Can you work these out from the model? Positions are in its coordinate system, mm. A direction names the side the tool comes from. Give positions to 0.01 mm unless a question says otherwise; leave off trailing zeros. Loops run counter-clockwise (first coordinate to the right, second up) from the corner with the lowest first, then second, coordinate; pieces in that order, holes last. Notation, with made-up numbers: (10.25, 71.5) - (58.25, 71.5) arc R11 cw to (58.25, 79.5) - close; hole circle Ø6 at (21.5, 24.25). An arc over 180 degrees is marked (long way). Answer in a Markdown table with one row per item.
Autodesk Inventor part; units mm, degrees
ref_plane "Work Plane1" through (0, 0, 10) normal (0, 0, 1) x (1, 0, 0)
ref_plane "YZ Plane" through (0, 0, 0) normal (1, 0, 0) x (0, 1, 0)
ref_plane "XZ Plane" through (0, 0, 0) normal (0, 1, 0) x (-1, 0, 0)
ref_plane "Work Plane1" through (0, 0, 10) normal (0, 0, 1) x (1, 0, 0)
sketch "Sketch1" plane through (0, 0, 10) normal (0, 0, 1) x (1, 0, 0)
  line L0 (-4.0299, -0.3538) -> (-2.2322, 1.4439) construction
  arc A0 (-1.4439, 2.2322) -> (-2.2322, 1.4439) centre (-0.9299, 0.9299) ccw construction
  line L1 (-1.4439, 2.2322) -> (0.3538, 4.0299) construction
  line L2 (-37.8299, 42.8299) -> (-37.8299, 37.8299) construction
  line L3 (-37.8299, 37.8299) -> (-42.9208, 37.8299) construction
  line L4 (-37.8299, 42.2137) -> (-37.8299, 45.8299) construction
  line L5 (-37.8299, 45.8299) -> (-4.0299, 45.8299) construction
  line L6 (-4.0299, 45.8299) -> (-4.0299, 42.2137) construction
  line L7 (-4.0299, 4.0299) -> (0.3538, 4.0299)
  circle A1 centre (-20.9299, 20.9299) radius 17.5
  line L8 (-20.9299, 58.9723) -> (17.1124, 20.9299) construction
  line L9 (17.1124, 20.9299) -> (-20.9299, -17.1124) construction
  line L10 (-20.9299, -17.1124) -> (-58.9723, 20.9299) construction
  line L11 (-58.9723, 20.9299) -> (-20.9299, 58.9723) construction
  line L12 (-20.9299, 58.9723) -> (-20.9299, -17.1124) construction
  line L13 (17.1124, 20.9299) -> (-58.9723, 20.9299) construction
  line L14 (-20.9299, 58.9723) -> (32.8701, 58.9723) construction
  line L15 (-43.4299, 43.4299) -> (1.5701, 43.4299) construction
  line L16 (1.5701, 43.4299) -> (1.5701, -1.5701) construction
  line L17 (1.5701, -1.5701) -> (-43.4299, -1.5701) construction
  line L18 (-43.4299, -1.5701) -> (-43.4299, 43.4299) construction
  line L19 (-43.4299, 43.4299) -> (1.5701, -1.5701) construction
  line L20 (1.5701, 43.4299) -> (-43.4299, -1.5701) construction
  line L21 (-43.4299, 5.3876) -> (-43.4299, 36.4723)
  line L22 (-43.4299, 36.4723) -> (-36.4723, 43.4299)
  line L23 (-36.4723, 43.4299) -> (-5.3876, 43.4299)
  line L24 (-5.3876, 43.4299) -> (1.5701, 36.4723)
  line L25 (1.5701, 36.4723) -> (1.5701, 5.3876)
  line L26 (1.5701, 5.3876) -> (-5.3876, -1.5701)
  line L27 (-5.3876, -1.5701) -> (-36.4723, -1.5701)
  line L28 (-36.4723, -1.5701) -> (-43.4299, 5.3876)
  line L29 (-4.0299, 42.2137) -> (-37.8299, 42.2137)
  line L30 (-4.0299, -0.3538) -> (-4.0299, 4.0299)
  circle A2 centre (-20.9299, 20.9299) radius 1.5
  line L31 (-10.9299, 10.9299) -> (-30.9299, 10.9299) construction
  line L32 (-30.9299, 10.9299) -> (-30.9299, 30.9299) construction
  line L33 (-30.9299, 30.9299) -> (-10.9299, 30.9299) construction
  line L34 (-10.9299, 30.9299) -> (-10.9299, 10.9299) construction
  line L35 (-10.9299, 10.9299) -> (-30.9299, 30.9299) construction
  line L36 (-30.9299, 10.9299) -> (-10.9299, 30.9299) construction
  circle A3 centre (-30.9299, 30.9299) radius 1.4
  circle A4 centre (-30.9299, 10.9299) radius 1.4
  circle A5 centre (-10.9299, 10.9299) radius 1.4
  line L37 (-45.8299, 37.8299) -> (-42.0723, 37.8299) construction
  line L38 (-42.1723, 37.7299) -> (-45.8299, 37.7299)
  line L39 (-45.8299, 37.7299) -> (-45.8299, 4.1299)
  line L40 (-45.8299, 4.1299) -> (-42.1723, 4.1299)
  line L41 (-42.1723, 4.1299) -> (-42.1723, 37.7299)
  line L42 (-45.8299, 4.0299) -> (-42.0723, 4.0299) construction
  line L43 (-45.8299, 37.8299) -> (-42.0723, 37.8299)
  line L44 (-37.7299, 45.8299) -> (-4.1299, 45.8299)
  line L45 (-4.1299, 45.8299) -> (-4.1299, 42.1723)
  line L46 (-4.1299, 42.1723) -> (-37.7299, 42.1723)
  line L47 (-37.7299, 42.1723) -> (-37.7299, 45.8299)
  line L48 (0.4701, 37.8299) -> (0.4701, 4.0299) construction
  line L49 (0.4701, 4.0299) -> (3.9701, 4.0299) construction
  line L50 (3.9701, 37.8299) -> (3.9701, 4.0299) construction
  line L51 (0.4701, 37.8299) -> (3.9701, 37.8299) construction
  line L52 (-45.8299, -3.9701) -> (-4.0299, -3.9701) construction
  line L53 (0.3124, 37.7299) -> (3.9701, 37.7299)
  line L54 (3.9701, 37.7299) -> (3.9701, 4.1299)
  line L55 (3.9701, 4.1299) -> (0.3124, 4.1299)
  line L56 (0.3124, 4.1299) -> (0.3124, 37.7299)
  line L57 (-4.1713, -0.3538) -> (-37.7299, -0.3538)
  line L58 (-37.7299, -0.3538) -> (-37.7299, -3.9701)
  line L59 (-37.7299, -3.9701) -> (-4.1713, -3.9701)
  line L60 (-4.1713, -3.9701) -> (-4.1713, -0.3538)
  point P0 (-37.8299, 4.0299)
  dimension "d18" = 53.8
  dimension "d19" = 45
  dimension "d20" = 53.8
  dimension "d21" = 45
  dimension "d22" = 45
  dimension "d30" = 20
  dimension "d31" = 20
  dimension "d32" = 2.8
  dimension "d33" = 2.8
  dimension "d34" = 2.8
  dimension "d35" = 3
  dimension "d36" = 0.1
  dimension "d37" = 0.1
  dimension "d38" = 0.1
  dimension "d39" = 0.1
extrude "Extrusion1" add sketch "Sketch1" along normal blind 3 contours L30 L26 L57 L28 L41 L22 L46 L24 L56 L7 | L7 L26 L30 | L56 L24 L25 L26 | L26 L25 L24 L53 L54 L55 | L60 L59 L58 L57 L28 L27 L26 | L26 L27 L28 L57 | L46 L22 L29 L24 | L24 L29 L45 | L40 L39 L38 L22 L21 L28 | L28 L21 L22 L41 | L29 L22 L23 L24 | L24 L23 L22 L29 L47 L44 L45 | L47 L29 L22 | A1 | A2 | A3 | A4 | A5
sketch "Skizze4" plane through (0, 0, 13) normal (0, 0, 1) x (1, 0, 0)
  line L0 (-37.7299, 42.1723) -> (-42.1723, 37.7299)
  line L1 (-42.1723, 37.7299) -> (-45.8299, 37.7299)
  line L2 (-45.8299, 37.7299) -> (-45.8299, 4.1299) construction
  line L3 (-45.8299, 4.1299) -> (-42.1723, 4.1299)
  line L4 (-42.1723, 4.1299) -> (-37.6885, -0.3538)
  line L5 (-37.6885, -0.3538) -> (-37.7299, -0.3538)
  line L6 (-37.7299, -0.3538) -> (-37.7299, -3.9701)
  line L7 (-37.7299, -3.9701) -> (-4.1713, -3.9701) construction
  line L8 (-4.1713, -3.9701) -> (-4.1713, -0.3538)
  line L9 (-4.1713, -0.3538) -> (0.3124, 4.1299)
  line L10 (0.3124, 4.1299) -> (3.9701, 4.1299)
  line L11 (3.9701, 4.1299) -> (3.9701, 37.7299) construction
  line L12 (3.9701, 37.7299) -> (0.3124, 37.7299)
  line L13 (0.3124, 37.7299) -> (-4.1299, 42.1723)
  line L14 (-4.1299, 42.1723) -> (-4.1299, 45.8299)
  line L15 (-4.1299, 45.8299) -> (-37.7299, 45.8299) construction
  line L16 (-37.7299, 45.8299) -> (-37.7299, 42.1723)
  line L17 (-37.9299, 46.0299) -> (-3.9299, 46.0299) construction
  line L18 (-3.9299, 46.0299) -> (-3.9299, 42.2551)
  line L19 (-3.9299, 42.2551) -> (0.3953, 37.9299)
  line L20 (0.3953, 37.9299) -> (4.1701, 37.9299)
  line L21 (4.1701, 37.9299) -> (4.1701, 3.9299) construction
  line L22 (4.1701, 3.9299) -> (0.3953, 3.9299)
  line L23 (0.3953, 3.9299) -> (-3.9713, -0.4367)
  line L24 (-3.9713, -0.4367) -> (-3.9713, -4.1701)
  line L25 (-3.9713, -4.1701) -> (-37.9299, -4.1701) construction
  line L26 (-37.9299, -4.1701) -> (-37.9299, -0.3953)
  line L27 (-37.9299, -0.3953) -> (-42.2551, 3.9299)
  line L28 (-42.2551, 3.9299) -> (-46.0299, 3.9299)
  line L29 (-46.0299, 3.9299) -> (-46.0299, 37.9299) construction
  line L30 (-46.0299, 37.9299) -> (-42.2551, 37.9299)
  line L31 (-42.2551, 37.9299) -> (-37.9299, 42.2551)
  line L32 (-37.9299, 42.2551) -> (-37.9299, 46.0299)
  line L33 (-45.8299, 37.7299) -> (-45.8299, 37.9299)
  line L34 (-4.1299, 45.8299) -> (-37.7299, 45.8299)
  line L35 (-37.7299, 45.8299) -> (-37.9299, 45.8299)
  line L36 (-4.1299, 45.8299) -> (-3.9299, 45.8299)
  line L37 (3.9701, 37.7299) -> (3.9701, 37.9299)
  line L38 (3.9701, 4.1299) -> (3.9701, 37.7299)
  line L39 (3.9701, 4.1299) -> (3.9701, 3.9299)
  line L40 (-4.1713, -3.9701) -> (-3.9713, -3.9701)
  line L41 (-37.7299, -3.9701) -> (-37.9299, -3.9701)
  line L42 (-45.8299, 4.1299) -> (-45.8299, 3.9299)
  point P0 (0, 0)
  dimension "d40" = 0.2
extrude "IM_offset" add sketch "Skizze4" against normal up to surface (3 mm away)
ref_plane "Arbeitsebene5" through (-20.9299, 3.9299, 10) normal (1, 0, 0) x (0, 0, -1)
ref_plane "Arbeitsebene6" through (-37.9299, 20.9299, 10) normal (0, 1, 0) x (1, 0, 0)
sketch "Skizze25" plane through (0, 0, 13) normal (0, 0, 1) x (1, 0, 0)
  line L0 (3.9701, 3.9299) -> (3.9701, 37.9299)
  line L1 (3.9701, 37.9299) -> (0.3953, 37.9299)
  line L2 (0.3953, 37.9299) -> (-3.9299, 42.2551)
  line L3 (-3.9299, 42.2551) -> (-3.9299, 45.8299)
  line L4 (-3.9299, 45.8299) -> (-37.9299, 45.8299)
  line L5 (-37.9299, 45.8299) -> (-37.9299, 42.2551)
  line L6 (-37.9299, 42.2551) -> (-42.2551, 37.9299)
  line L7 (-42.2551, 37.9299) -> (-45.8299, 37.9299)
  line L8 (-45.8299, 37.9299) -> (-45.8299, 3.9299)
  line L9 (-42.2551, 3.9299) -> (-45.8299, 3.9299)
  line L10 (-37.9299, -0.3953) -> (-42.2551, 3.9299)
  line L11 (-37.9299, -3.9701) -> (-37.9299, -0.3953)
  line L12 (-3.9713, -3.9701) -> (-37.9299, -3.9701)
  line L13 (-3.9713, -3.9701) -> (-3.9713, -0.4367)
  line L14 (-3.9713, -0.4367) -> (0.3953, 3.9299)
  line L15 (0.3953, 3.9299) -> (3.9701, 3.9299)
  line L16 (-11.384, 9.2627) -> (-32.5972, 30.4759)
  line L17 (-15.9506, 25.9092) -> (-25.9506, 25.9092)
  line L18 (-25.9506, 25.9092) -> (-25.9506, 15.9092)
  line L19 (-25.9506, 15.9092) -> (-15.9506, 15.9092)
  line L20 (-15.9506, 15.9092) -> (-15.9506, 25.9092)
  line L21 (-15.9506, 25.9092) -> (-25.9506, 15.9092) construction
  line L22 (-25.9506, 25.9092) -> (-15.9506, 15.9092) construction
  line L23 (-13.9506, 27.9092) -> (-27.9506, 27.9092)
  line L24 (-27.9506, 27.9092) -> (-27.9506, 13.9092)
  line L25 (-27.9506, 13.9092) -> (-13.9506, 13.9092)
  line L26 (-13.9506, 13.9092) -> (-13.9506, 27.9092)
  line L27 (-15.9506, 20.9092) -> (-13.9506, 20.9092)
  line L28 (-20.9506, 25.9092) -> (-20.9506, 27.9092)
  line L29 (-18.0305, 15.9092) -> (-15.9506, 18.072)
  line L30 (-25.9506, 23.8293) -> (-23.7879, 25.9092)
  line L31 (-27.9506, 27.9092) -> (-25.9506, 27.9092)
  line L32 (-13.9506, 13.9092) -> (-8.2901, 13.9092)
  line L33 (-8.2901, 13.9092) -> (-8.2901, 15.9092)
  line L34 (-8.2901, 15.9092) -> (-13.9506, 15.9092)
  line L35 (-13.9506, 15.9092) -> (-13.9506, 13.9092)
  line L36 (-8.2901, 15.9092) -> (-13.9506, 21.5697)
  point P0 (0, 0)
  point P1 (-20.9506, 20.9092)
  point P2 (-13.9506, 15.9092)
  dimension "d150" = 10
  dimension "d151" = 10
  dimension "d152" = 2
  dimension "d154" = 7
extrude "Extrusion21" add sketch "Skizze25" along normal blind 25 contours L19 L20 L27 L26 L25 L16 | L16 L25 L24 L18 L19 | L16 L24 L23 L28 L17 L18 | L26 L34 L33 L32 | L20 L17 L28 L23 L26 L27 | L26 L36 L34
ref_plane "Arbeitsebene10" through (0, 0, 42) normal (0, 0, 1) x (1, 0, 0)
ref_plane "Arbeitsebene9" through (-28.9506, 12.9092, 13) normal (-1, 0, 0) x (0, 0, 1)
sketch "Skizze28" plane through (-28.9506, 12.9092, 13) normal (-1, 0, 0) x (0, 0, 1)
  line L0 (0, 3) -> (0, 13)
  line L1 (0, 3) -> (25, 3)
  line L2 (25, 13) -> (25, 3)
  line L3 (0, 13) -> (25, 13)
  line L4 (17.5, 3) -> (7.5, 3)
  line L5 (7.5, 3) -> (7.5, 6)
  line L6 (7.5, 6) -> (17.5, 6)
  line L7 (17.5, 6) -> (17.5, 3)
  line L8 (17.5, 3) -> (7.5, 6) construction
  line L9 (7.5, 3) -> (17.5, 6) construction
  point P0 (-13, -12.9092)
  point P1 (12.5, 4.5)
  point P2 (17.5, 3)
  point P3 (17.5, 13)
  point P4 (7.5, 13)
  dimension "d187" = 10
  dimension "d188" = 3
extrude "Extrusion24" cut sketch "Skizze28" against normal blind 3 contours L5 L6 L7 L1
sketch "Skizze34" plane through (-27.9506, 13.9092, 13) normal (0, -1, 0) x (1, 0, 0)
  line L0 (19.6605, 0) -> (0, 0)
  line L1 (19.6605, 0) -> (19.6605, 25)
  line L2 (0, 25) -> (19.6605, 25)
  line L3 (0, 0) -> (0, 25)
  circle A0 centre (8.0421, 12.5) radius 5.5
  point P0 (27.9506, -13)
  dimension "d192" = 11
extrude "Extrusion30" cut sketch "Skizze34" against normal blind 3 contours A0
sketch "Skizze35" plane through (-27.9506, 13.9092, 13) normal (0, -1, 0) x (1, 0, 0)
  circle A0 centre (8.0421, 12.5) radius 5.5
  circle A1 centre (8.0421, 12.5) radius 6.5
  point P0 (27.9506, -13)
  dimension "d195" = 13
extrude "Extrusion31" cut sketch "Skizze35" against normal blind 1 contours A0 | A1
sketch "Skizze36" plane through (-27.9506, 13.9092, 13) normal (-1, 0, 0) x (0, 0, 1)
  circle A0 centre (12.5608, 1.7467) radius 6.5
  point P0 (-13, -13.9092)
  dimension "d202" = 13
extrude "Extrusion32" cut sketch "Skizze36" against normal blind 1
ref_plane "Arbeitsebene12" through (-8.2901, 13.9092, 13) normal (0.9063, -0.4226, 0) x (0, 0, 1)
sketch "Skizze37" plane through (-8.2901, 13.9092, 13) normal (0.9063, -0.4226, 0) x (0, 0, 1)
  circle A0 centre (12.5, -0.6497) radius 1
  ellipse E0 centre (12.5, 4.9101) end of major axis (6, 4.9101) minor radius 2.747
  point P0 (-13, 9.1025)
  dimension "d204" = 2
extrude "Extrusion33" cut sketch "Skizze37" against normal through all contours A0
properties part number "20_Cube_Insert_Lightsheet_FEPTube_Flowcube_small_v3"
Q1. Imagine slicing it at B-B, the plane z = 33.25. Write out the boundary of the cut face in (x, y).
Checked values:
| item | result |
|---|---|
| outline | (-27.95, 13.91) - (-8.29, 13.91) - (-8.29, 15.91) - (-13.95, 21.57) - (-13.95, 27.91) - (-27.95, 27.91) - close; hole (-25.95, 15.91) - (-15.95, 15.91) - (-15.95, 25.91) - (-25.95, 25.91) - close |
Q2. Imagine slicing it at D-D, the plane x = -7. Write out the boundary of the cut face in (y, z).
Checked values:
| item | result |
|---|---|
| outline | (-3.97, 10) - (45.83, 10) - (45.83, 13) - (-3.97, 13) - close |
Q3. Imagine slicing it at C-C, the plane z = 12.25. Write out the boundary of the cut face in (x, y), and give its area (3 significant figures).
Checked values:
| item | result |
|---|---|
| outline | (-45.83, 3.93) - (-42.26, 3.93) - (-37.93, -0.4) - (-37.93, -3.97) - (-3.97, -3.97) - (-3.97, -0.44) - (0.4, 3.93) - (3.97, 3.93) - (3.97, 37.93) - (0.4, 37.93) - (-3.93, 42.26) - (-3.93, 45.83) - (-37.93, 45.83) - (-37.93, 42.26) - (-42.26, 37.93) - (-45.83, 37.93) - close |
| area | 2,270 mm² |
Q4. Imagine slicing it at A-A, the plane z = 25.5. Count the separate pieces of the cut face and the enclosed holes in it, and give its area (3 significant figures).
Checked values:
| item | result |
|---|---|
| separate pieces | 5 |
| enclosed holes | 0 |
| area | 65.7 mm² |
Q5. If I drill on line 1 (Y direction, x = -17, z = 15); line 2 (X direction, y = 25, z = 25.75); line 3 (Z direction, x = -40, y = 6.5), over which ranges is the centre line in solid material (lowest first)? Write a range as [from, to].
Checked values:
| item | result |
|---|---|
| line 1 | y = [13.91, 15.91], [25.91, 27.91] |
| line 2 | x = [-27.95, -25.95], [-15.95, -13.95] |
| line 3 | z = [10, 13] |
Q6. On a 3-axis mill with a long thin cutter (end or side, diameter ignored), from which of +Z, -Z, +X, -X, +Y, -Y can I reach the whole of each face in a straight line? I mean faces 4 (the face through (-13.951, 25, 25)), 5 (the face through (-37.93, -2, 12)), 6 (the face through (-8.29, 15, 23)). Say none if no direction works.
Checked values:
| item | result |
|---|---|
| face 4 | +Z, +X, +Y |
| face 5 | +Z, -Z, -X, -Y |
| face 6 | +Z, +X, +Y, -Y |
Q7. If we mould it in two halves opening along Y, with no side actions, what happens to faces 1 (the face through (-21, 21, 13)), 2 (the face through (-45.83, 21, 11)), 3 (the face through (-21, -3.97, 11))? For each: released by +Y, released by -Y, zero draft, split by the parting line, or undercut.
Checked values:
| item | result |
|---|---|
| face 1 | undercut |
| face 2 | zero draft |
| face 3 | released by -Y |
Q8. For pin 1 (3 mm diameter, centred on y = 25.5, z = 20.5, fed in from +X); pin 2 (6 mm diameter, centred on x = -33, z = 31.5, fed in from +Y); pin 3 (1.5 mm diameter, centred on x = -44, z = 11.5, fed in from -Y); pin 4 (1 mm diameter, centred on x = -22, z = 18, fed in from +Y), each with a flat end and sliding along its axis, tell me the tip position at first contact or that it passes through.
Checked values:
| item | result |
|---|---|
| pin 1 | stops at x = -13.95 |
| pin 2 | passes through |
| pin 3 | stops at y = 3.93 |
| pin 4 | stops at y = 27.91 |
